Build history of the part. All positions in model axes, mm. A direction names the side the tool comes from. Round coordinates to 2 decimals unless told otherwise and drop trailing zeros. Loops run counter-clockwise (first coordinate to the right, second up) from the corner with the lowest first, then second, coordinate; pieces in that order, holes last. Notation, with made-up numbers: M 3.25,51.5 L 15.25,51.5 A33 ccw 15.25,86.5 Z; hole C 16.25,79.25 d5. An arc over 180 degrees is marked long. One line per item, written item: value.
```python
from build123d import *

# Parameters (mm, degrees)
BOSS_EXTRUDE1_DEPTH   = 2
M3_TAPPED_HOLE1_D     = 2.5
M3_TAPPED_HOLE1_DEPTH = 7.5
M3_TAPPED_HOLE1_TIP   = 0.751075774
SKETCH5_R             = 4
CUT_EXTRUDE4_DEPTH    = 0.6


with BuildPart() as part:
    # Sketch1 → Boss-Extrude1 (new body)
    with BuildSketch(Plane.XY.offset(3.579115056)):
        with BuildLine():
            Line((13.461651474, 21.151347876), (-19.538348526, 21.151347876))
            ThreePointArc((-19.538348526, 21.151347876), (-21.447536835, 20.360536186), (-22.238348526, 18.451347876))
            Line((-22.238348526, 18.451347876), (-22.238348526, -27.548652124))
            ThreePointArc((-22.238348526, -27.548652124), (-21.447536835, -29.457840433), (-19.538348526, -30.248652124))
            Line((-19.538348526, -30.248652124), (13.461651474, -30.248652124))
            ThreePointArc((13.461651474, -30.248652124), (15.370839783, -29.457840433), (16.161651474, -27.548652124))
            Line((16.161651474, -27.548652124), (16.161651474, 18.451347876))
            ThreePointArc((16.161651474, 18.451347876), (15.370839783, 20.360536186), (13.461651474, 21.151347876))
        make_face()
    extrude(amount=BOSS_EXTRUDE1_DEPTH)

    # M3 Tapped Hole1
    with Locations(Plane(origin=(0, 0, 3.579115056), x_dir=(-1, 0, 0), z_dir=(0, 0, -1))):
        with Locations((19.538348526, 18.451347876), (-13.461651474, 18.451347876), (-13.461651474, -27.548652124), (19.538348526, -27.548652124)):
            Hole(M3_TAPPED_HOLE1_D / 2, depth=M3_TAPPED_HOLE1_DEPTH)
            with Locations((0, 0, -(M3_TAPPED_HOLE1_DEPTH + M3_TAPPED_HOLE1_TIP / 2))):  # 118° drill point
                Cone(0, M3_TAPPED_HOLE1_D / 2, M3_TAPPED_HOLE1_TIP, mode=Mode.SUBTRACT)

    # Sketch5 → Cut-Extrude4 (cut)
    with BuildSketch(Plane(origin=(0, 0, 3.579115056), x_dir=(-1, 0, 0), z_dir=(0, 0, -1))):
        with Locations((3.038348526, 4.451347876)):
            Circle(SKETCH5_R)
    extrude(amount=-CUT_EXTRUDE4_DEPTH, mode=Mode.SUBTRACT)


solid = part.part
```
Item 1: Which spindle directions (+Z, -Z, +X, -X, +Y, -Y) get a long thin tool onto all of the face, cutting with end or side? Do faces 4 (the face through (15.35, -29.48, 4.57)), 5 (the face through (-2.171, 0.546, 3.875)). Say none if no direction does.
Check values:
face 4: +Z, -Z, +X, -Y
face 5: -Z
Item 2: Pull direction X, two halves, no side cores. Call faces 1 (the face through (-22.238, -4, 5)), 2 (the face through (16.162, -5, 5)), 3 (the face through (-3, 5, 4.179)): pulls with the +X half, pulls with the -X half, needs draft (parallel to the pull), parting line crosses it, or undercut.
Check values:
face 1: pulls with the -X half
face 2: pulls with the +X half
face 3: undercut
Item 3: Slice it at A-A, the plane y = 7. Give the cut face in (x, z), and give its area (3 significant figures).
Check values:
outline: M -22.24,3.58 L -6.12,3.58 L -6.12,4.18 L 0.04,4.18 L 0.04,3.58 L 16.16,3.58 L 16.16,5.58 L -22.24,5.58 Z
area: 73.1 mm2
Item 4: Drop flat-ended pins along their axis: P1, Ø2, axis at x = -19.54, y = -27.55, coming from the +Z side; P2, Ø6.5, axis at x = -2.5, y = 6, coming from the -Z side. Give the stop position or say it passes through.
Check values:
P1: passes through
P2: stops at z = 3.58
Item 5: Slice it at B-B, the plane x = -3. Give the cut face in (y, z).
Check values:
outline: M -30.25,3.58 L 0.45,3.58 L 0.45,4.18 L 8.45,4.18 L 8.45,3.58 L 21.15,3.58 L 21.15,5.58 L -30.25,5.58 Z
